Geometry: final body of the model. Coordinates: model frame, mm. A direction names the side the tool comes from. Round coordinates to 2 decimals unless told otherwise and drop trailing zeros. Loops run counter-clockwise (first coordinate to the right, second up) from the corner with the lowest first, then second, coordinate; pieces in that order, holes last. Notation, with made-up numbers: (-11.75, 60.25) -> (46.25, 60.25) arc R3 cw to (46.25, 65.25) -> close; hole circle Ø10 at (60.5, -2.75). An arc over 180 degrees is marked (long way). Answer in a Markdown table with one row per item.
Autodesk Inventor part; units mm, degrees
ref_plane "YZ Plane" through (0, 0, 0) normal (1, 0, 0) x (0, 1, 0)
ref_plane "XZ Plane" through (0, 0, 0) normal (0, 1, 0) x (-1, 0, 0)
ref_plane "XY Plane" through (0, 0, 0) normal (0, 0, 1) x (1, 0, 0)
sketch "Эскиз1" plane through (0, 0, 0) normal (0, 0, 1) x (1, 0, 0)
  line L0 (-4, -1) -> (4, -1)
  line L1 (4, -1) -> (4, 1)
  line L2 (4, 1) -> (-4, 1)
  line L3 (-4, 1) -> (-4, -1)
  line L4 (-4, -1) -> (4, 1) construction
  line L5 (4, -1) -> (-4, 1) construction
  point P0 (0, 0)
  dimension "d0" = 8
  dimension "d1" = 2
extrude "Выдавливание1" add sketch "Эскиз1" along normal blind 5
sketch "Эскиз2" plane through (-4, 1, 0) normal (0, 1, 0) x (1, 0, 0)
  line L0 (0, 0) -> (0, -5)
  circle A0 centre (0, -2.5) radius 2.5
  line L1 (8, 0) -> (8, -5)
  circle A1 centre (8, -2.5) radius 2.5
  point P0 (4, 0)
  dimension "d4" = 5
  dimension "d5" = 5
extrude "Выдавливание2" add sketch "Эскиз2" against normal blind 2
sketch "Эскиз3" plane through (-4, 1, 0) normal (0, 1, 0) x (1, 0, 0)
  arc A0 (0, 0) -> (0, -5) centre (0, -2.5) ccw
  circle A1 centre (0, -2.5) radius 0.75
  arc A2 (8, -5) -> (8, 0) centre (8, -2.5) ccw
  circle A3 centre (8, -2.5) radius 0.75
  point P0 (4, 0)
  dimension "d8" = 1.5
  dimension "d9" = 1.5
extrude "Выдавливание3" cut sketch "Эскиз3" against normal blind 2
sketch "Эскиз4" plane through (-4, 1, 0) normal (0, 1, 0) x (1, 0, 0)
  line L0 (4, 0) -> (4, -5)
  line L1 (0, -5) -> (8, -5)
  line L2 (0, 0) -> (8, 0)
  line L3 (6.9421, -5) -> (0.9421, -5)
  line L4 (0.9421, -5) -> (0.9421, 0)
  line L5 (0.9421, 0) -> (6.9421, 0)
  line L6 (6.9421, 0) -> (6.9421, -5)
  line L7 (6.9421, -5) -> (0.9421, 0) construction
  line L8 (0.9421, -5) -> (6.9421, 0) construction
  point P0 (3.9421, -2.5)
  dimension "d12" = 6
extrude "Выдавливание4" cut sketch "Эскиз4" against normal blind 1
sketch "Эскиз5" plane through (0, 0, 0) normal (0, 0, -1) x (-1, 0, 0)
  line L0 (-3.25, -1) -> (-4.75, -1)
  line L1 (-4, -1) -> (4, -1)
  line L2 (4, -1) -> (4, 3)
  line L3 (4, 3) -> (-4, 3)
  line L4 (-4, 3) -> (-4, -1)
  point P0 (0, 0)
  dimension "d15" = 8
  dimension "d16" = 4
extrude "Выдавливание5" add sketch "Эскиз5" along normal blind 2
sketch "Эскиз6" plane through (0, 0, -2) normal (0, 0, -1) x (-1, 0, 0)
  line L0 (-4, 3) -> (-4, 1)
  line L1 (-4, 1) -> (4, 1)
  line L2 (3.25, 1) -> (4.75, 1)
  circle A0 centre (0, 1) radius 0.75
  circle A1 centre (0, 1) radius 1.6
  point P0 (0, 0)
  dimension "d19" = 1.5
  dimension "d20" = 3.2
extrude "Выдавливание6" add sketch "Эскиз6" along normal blind 2 contours A0 L1 A1 | L1 A1 A0
sketch "Эскиз7" plane through (-4, 1, 5) normal (0, 1, 0) x (1, 0, 0)
  circle A0 centre (0, 2.5) radius 0.75
  line L0 (0.9421, 0) -> (0.9421, 5)
  line L1 (0.9421, 5) -> (0, 5)
  arc A1 (0, 5) -> (0, 0) centre (0, 2.5) ccw
  line L2 (0.9421, 0) -> (0, 0)
  line L3 (0.9421, 0) -> (0.9421, 5)
  line L4 (6.9421, 0) -> (0.9421, 0)
  line L5 (6.9421, 5) -> (6.9421, 0)
  line L6 (0.9421, 5) -> (6.9421, 5)
  circle A2 centre (8, 2.5) radius 0.75
  line L7 (6.9421, 5) -> (6.9421, 0)
  line L8 (8, 0) -> (6.9421, 0)
  arc A3 (8, 0) -> (8, 5) centre (8, 2.5) ccw
  line L9 (8, 5) -> (6.9421, 5)
  point P0 (4, 5)
properties part number "КВ33.044.206 - Крепеж держателя ремня" material "Пластик АБС"
Item 1: Reachability of faces 1 (the face through (-6.5, 0, 2.4)), 2 (the face through (-5, 1, 2)), 3 (the face through (0.098, 0.256, -2.986)), 4 (the face through (6.5, 0, 2.6)), 5 (the face through (-4, 1, -1)) from +Z, -Z, +X, -X, +Y, -Y: full face, straight path, thin tool, end or side. Return the list, or none.
Answer:
| item | result |
|---|---|
| face 1 | -X, +Y, -Y |
| face 2 | +Z, +X, -X, +Y |
| face 3 | -Z |
| face 4 | +X, +Y, -Y |
| face 5 | -Z, -X, +Y, -Y |
Item 2: Draft query along X for faces 6 (the face through (-1, 1, -4)), 7 (the face through (4, 1, -1)), 8 (the face through (0, 0, 2)), 9 (the face through (2.942, 0.5, 2.5)). Return one class per face: pulls with the +X half, pulls with the -X half, needs draft (parallel to the pull), parting line crosses it, or undercut.
Answer:
| item | result |
|---|---|
| face 6 | needs draft |
| face 7 | pulls with the +X half |
| face 8 | undercut |
| face 9 | undercut |
Item 3: Cut plane D-D (z = -1.75). Output: boundary loops of the cut face in (x, y), then the cut area to 3 significant figures.
Answer:
| item | result |
|---|---|
| outline | (-4, -1) -> (4, -1) -> (4, 3) -> (-4, 3) -> close |
| area | 32.0 mm² |
Item 4: Line query: probe 1 along X at (y, z) = (0.35, 2.5); probe 2 along X at (y, z) = (-0.5, 2.5); probe 3 along X at (y, z) = (1, -2.7). Output: solid intervals per line, ascending. Write a range as [from, to].
Answer:
| item | result |
|---|---|
| probe 1 | x = [-6.5, -4.75], [-3.25, -3.06], [2.94, 3.25], [4.75, 6.5] |
| probe 2 | x = [-6.5, -4.75], [-3.25, 3.25], [4.75, 6.5] |
| probe 3 | x = [-1.6, -0.75], [0.75, 1.6] |
Item 5: Cut plane B-B (x = -2.75). Output: boundary loops of the cut face in (y, z).
Answer:
| item | result |
|---|---|
| outline | (-1, -2) -> (3, -2) -> (3, 0) -> (0, 0) -> (0, 5) -> (-1, 5) -> close |
Item 6: Pin query (flat end, axial travel): pin 1 Ø1.5 at (x, y) = (-1.5, 1) entering from +Z; pin 2 Ø1.1 at (x, z) = (5, 3.5) entering from +Y; pin 3 Ø1.1 at (y, z) = (0.5, 1.5) entering from +X. Return the tip coordinate at first contact, or that it passes through.
Answer:
| item | result |
|---|---|
| pin 1 | stops at z = 0 |
| pin 2 | stops at y = 1 |
| pin 3 | stops at x = 6.46 |
Item 7: Cut plane C-C (y = 2.4). Output: boundary loops of the cut face in (x, z).
Answer:
| item | result |
|---|---|
| outline | (-4, -2) -> (-0.77, -2) -> (-0.77, -4) -> (0.77, -4) -> (0.77, -2) -> (4, -2) -> (4, 0) -> (-4, 0) -> close |
Item 8: Cut plane A-A (z = 2.5). Output: boundary loops of the cut face in (x, y), then the cut area to 3 significant figures.
Answer:
| item | result |
|---|---|
| outline | (-6.5, -1) -> (-4.75, -1) -> (-4.75, 1) -> (-6.5, 1) -> close; (-3.25, -1) -> (3.25, -1) -> (3.25, 1) -> (2.94, 1) -> (2.94, 0) -> (-3.06, 0) -> (-3.06, 1) -> (-3.25, 1) -> close; (4.75, -1) -> (6.5, -1) -> (6.5, 1) -> (4.75, 1) -> close |
| area | 14.0 mm² |
